```python
from build123d import *

# Parameters (mm, degrees)
BOSS_EXTRUDE1_DEPTH = 6
BOSS_EXTRUDE2_DEPTH = 6


with BuildPart() as part:
    # Sketch1 → Boss-Extrude1 (new body)
    with BuildSketch(Plane.XY):
        with BuildLine():
            Line((-49.804736885, 16.53410644), (-49.804736885, -371.46589356))
            ThreePointArc((-49.804736885, -371.46589356), (-48.340270791, -375.001427466), (-44.804736885, -376.46589356))
            Line((-44.804736885, -376.46589356), (243.195263115, -376.46589356))
            ThreePointArc((243.195263115, -376.46589356), (246.730797021, -375.001427466), (248.195263115, -371.46589356))
            Line((248.195263115, -371.46589356), (248.195263115, 16.53410644))
            ThreePointArc((248.195263115, 16.53410644), (246.730797021, 20.069640346), (243.195263115, 21.53410644))
            Line((243.195263115, 21.53410644), (-44.804736885, 21.53410644))
            ThreePointArc((-44.804736885, 21.53410644), (-48.340270791, 20.069640346), (-49.804736885, 16.53410644))
        make_face()
    extrude(amount=BOSS_EXTRUDE1_DEPTH)

    # Sketch2 → Boss-Extrude2 (add)
    with BuildSketch(Plane.XY.offset(6)):
        with BuildLine():
            Line((-39.804736885, 6.53410644), (-39.804736885, -361.46589356))
            ThreePointArc((-39.804736885, -361.46589356), (-38.340270791, -365.001427466), (-34.804736885, -366.46589356))
            Line((-34.804736885, -366.46589356), (233.195263115, -366.46589356))
            ThreePointArc((233.195263115, -366.46589356), (236.730797021, -365.001427466), (238.195263115, -361.46589356))
            Line((238.195263115, -361.46589356), (238.195263115, 6.53410644))
            ThreePointArc((238.195263115, 6.53410644), (236.730797021, 10.069640346), (233.195263115, 11.53410644))
            Line((233.195263115, 11.53410644), (-34.804736885, 11.53410644))
            ThreePointArc((-34.804736885, 11.53410644), (-38.340270791, 10.069640346), (-39.804736885, 6.53410644))
        make_face()
    extrude(amount=BOSS_EXTRUDE2_DEPTH)


solid = part.part
```
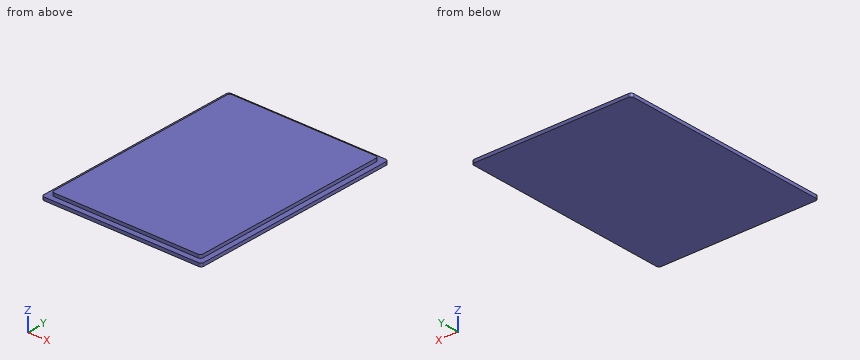
Geometry check sheet. Reference: the model listing, model coordinates, mm. Coordinates: 2 decimals unless noted, no trailing zeros. Write each loop counter-clockwise with the first axis right and the second up, starting at its lowest first coordinate (ties: lowest second). Pieces come first, ordered by that corner, then holes. Notation, with made-up numbers: (0.5, 74) -> (6.5, 74) arc R26 cw to (6.5, 97) -> close; hole circle Ø5 at (2.5, 83). An arc over 180 degrees is marked (long way). Use CSV: the item, a comma, the result in double quotes. Start each with the question number.
Item 1: Depth check by flat-ended pin: pin 1 Ø1.8 at (x, z) = (69, 10) entering from +Y; pin 2 Ø1.8 at (x, z) = (81, 8.5) entering from -Y; pin 3 Ø1 at (y, z) = (-306, 10.5) entering from -X. Enter the tip coordinate at first touch or a pass-through.
Item 2: Cross-section at A-A, the plane y = -177.5. Record the cut outline in (x, z).
Item 3: Thickness scan on line 1 (X direction, y = -68, z = 8.5); line 2 (Y direction, x = 132, z = 8.75). Record the ranges inside material, lowest first.
Item 4: Cross-section at B-B, the plane x = 39.5. Record the cut outline in (y, z), plus the area to 3 significant figures.
Answers:
1,pin 1,"y = 11.53"
1,pin 2,"y = -366.47"
1,pin 3,"x = -39.8"
2,outline,"(-49.8, 0) -> (248.2, 0) -> (248.2, 6) -> (238.2, 6) -> (238.2, 12) -> (-39.8, 12) -> (-39.8, 6) -> (-49.8, 6) -> close"
3,line 1,"-39.8 to 238.2"
3,line 2,"-366.47 to 11.53"
4,outline,"(-376.47, 0) -> (21.53, 0) -> (21.53, 6) -> (11.53, 6) -> (11.53, 12) -> (-366.47, 12) -> (-366.47, 6) -> (-376.47, 6) -> close"
4,area,"4,660 mm^2"
